from build123d import *

# Parameters (mm, degrees)
BOSS_EXTRUDE1_DEPTH = 152.4
SKETCH2_R           = 1.6
CUT_EXTRUDE1_DEPTH  = 0.1778
CUT_EXTRUDE4_DEPTH  = 152.0444
SKETCH6_R           = 1.6
CUT_EXTRUDE5_DEPTH  = 0.1778


with BuildPart() as part:
    # Sketch1 → Boss-Extrude1 (new body)
    with BuildSketch(Plane(origin=(0, 0, 0), x_dir=(0, 0, -1), z_dir=(1, 0, 0))):
        Polygon((43.890597967, 11.483842091), (31.890597967, 32.268451781), (22.25, 38.538130468), (44.5, 0), align=None)
        Polygon((22.25, 38.538130468), (44.5, 0), (0, 0), align=None)
        Polygon((0.609402033, 11.483842091), (12.609402033, 32.268451781), (22.25, 38.538130468), (0, 0), align=None)
        Polygon((10.25, -5.214163404), (34.25, -5.214163404), (44.5, 0), (0, 0), align=None)
    extrude(amount=BOSS_EXTRUDE1_DEPTH)

    # Sketch2 → Cut-Extrude1 (cut)
    with BuildSketch(Plane(origin=(152.4, 0, 0), x_dir=(0, 0, -1), z_dir=(1, 0, 0))):
        with Locations((22.25, 27.538130468)):
            Circle(SKETCH2_R)
        with Locations((34.973720558, 20.192086979)):
            Circle(SKETCH2_R)
        with Locations((34.973720558, 5.5)):
            Circle(SKETCH2_R)
        with Locations((22.25, -1.846043489)):
            Circle(SKETCH2_R)
        with Locations((9.526279442, 5.5)):
            Circle(SKETCH2_R)
        with Locations((9.526279442, 20.192086979)):
            Circle(SKETCH2_R)
        Polygon((16.441736842, 22.906250383), (10.633473684, 12.846043489), (16.441736842, 2.785836596), (28.058263158, 2.785836596), (33.866526316, 12.846043489), (28.058263158, 22.906250383), align=None)
    extrude(amount=-CUT_EXTRUDE1_DEPTH, mode=Mode.SUBTRACT)

    # Sketch4 → Cut-Extrude4 (cut)
    with BuildSketch(Plane(origin=(152.2222, 0, 0), x_dir=(0, 0, -1), z_dir=(1, 0, 0))):
        Polygon((22.25, 36.038130468), (2.165063509, 1.25), (42.334936491, 1.25), align=None)
    extrude(amount=-CUT_EXTRUDE4_DEPTH, mode=Mode.SUBTRACT)

    # Sketch6 → Cut-Extrude5 (cut)
    with BuildSketch(Plane.ZY):
        with Locations((-29.964101615, 17.299782134)):
            Circle(SKETCH6_R)
        with Locations((-14.535898385, 17.299782134)):
            Circle(SKETCH6_R)
        with Locations((-22.25, 3.938566201)):
            Circle(SKETCH6_R)
        Polygon((-22.25, 22.660998066), (-30.75, 7.938566201), (-13.75, 7.938566201), align=None)
    extrude(amount=-CUT_EXTRUDE5_DEPTH, mode=Mode.SUBTRACT)


solid = part.part
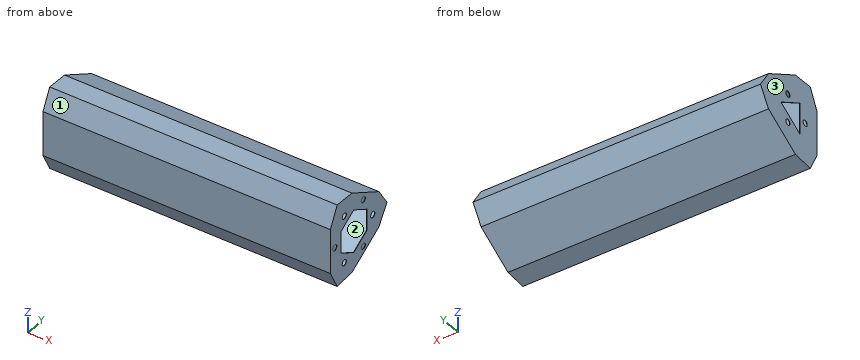
Can you work these out from the model? Positions are in its coordinate system, mm. Face numbers are marked on the shaded views. Give positions to 0.01 mm unless a question says otherwise; leave off trailing zeros. Loops run counter-clockwise (first coordinate to the right, second up) from the corner with the lowest first, then second, coordinate; pieces in that order, holes last. Notation, with made-up numbers: (26, 84) - (32, 84) arc R20 ccw to (32, 106) - close; hole circle Ø5 at (88, 11.25). An arc over 180 degrees is marked (long way). One line per item, written item: value.
(1) If we section it at C-C, the plane z = -18: List the corners of the cut face in (x, y) for me.
Verdict:
outline: (0, -5.21) - (152.4, -5.21) - (152.4, 2.79) - (152.22, 2.79) - (152.22, 1.25) - (0.18, 1.25) - (0.18, 7.94) - (0, 7.94) - close; (0, 15.3) - (0.18, 15.3) - (0.18, 28.68) - (152.22, 28.68) - (152.22, 22.91) - (152.4, 22.91) - (152.4, 35.77) - (0, 35.77) - close
(2) If we section it at A-A, the plane z = -26: List the corners of the cut face in (x, y) for me, plus the area to 3 significant figures.
Verdict:
outline: (0, -5.21) - (152.4, -5.21) - (152.4, 2.79) - (152.22, 2.79) - (152.22, 1.25) - (0.18, 1.25) - (0.18, 7.94) - (0, 7.94) - close; (0, 16.17) - (0.18, 16.17) - (0.18, 29.54) - (152.22, 29.54) - (152.22, 22.91) - (152.4, 22.91) - (152.4, 36.1) - (0, 36.1) - close
area: 1,990 mm^2
(3) If we mould it in two halves opening along X, with no side actions, what happens to the marked faces 1, 2 and 3? For each: released by +X, released by -X, zero draft, split by the parting line, or undercut.
Verdict:
face 1: zero draft
face 2: undercut
face 3: released by -X
(4) I need wall thicknesses on line 1 along Y through (x, z) = (0.05, -22.25); line 2 along X through (y, z) = (10.5, -31); line 3 along X through (y, z) = (25, -25). Which ranges of each line are inside material? Lowest first, please.
Verdict:
line 1: -5.21 to 2.34, 5.54 to 7.94, 22.66 to 38.54
line 2: 0 to 0.18
line 3: 0 to 0.18, 152.22 to 152.4
(5) If we section it at B-B, the plane x = 47: List the corners of the cut face in (y, z) for me.
Verdict:
outline: (-5.21, -34.25) - (0, -44.5) - (11.48, -43.89) - (32.27, -31.89) - (38.54, -22.25) - (32.27, -12.61) - (11.48, -0.61) - (0, 0) - (-5.21, -10.25) - close; hole (1.25, -42.33) - (36.04, -22.25) - (1.25, -2.17) - close
(6) I'm going to push flat-ended pins straight in: pin 1 (10.5 mm diameter, centred on y = 16, z = -21, fed in from +X); pin 2 (2 mm diameter, centred on x = 78.5, y = 34, fed in from +Z); pin 3 (10 mm diameter, centred on x = 81.5, y = 12, fed in from +Z). Where does each tip first touch, or does it pass through?
Verdict:
pin 1: x = 0.18
pin 2: z = -13.73
pin 3: z = -0.37
